from build123d import *

# Parameters (mm, degrees)
BOSS_EXTRUDE1_DEPTH     = 18
SKETCH2_R               = 3.175
CUT_EXTRUDE1_DEPTH      = 1.048172096
CUT_EXTRUDE1_DEPTH_BACK = 29.412494693
FILLET1_R               = 2.54


with BuildPart() as part:
    # Sketch1 → Boss-Extrude1 (new body)
    with BuildSketch(Plane.XY):
        with BuildLine():
            Line((0, -26.9), (25.314659544, -26.9))
            add(Edge.make_bspline(
                [(25.314659544, -26.9), (29.018808902, -26.95946599), (36.438320652, -26.653818936), (47.452273732, -24.92488313), (58.262486614, -21.924318782), (67.016013602, -18.37965694), (73.811742851, -14.890308818), (80.427413207, -11.130302547), (86.897235914, -7.369109823), (93.386399422, -4.327041649), (98.298472606, -2.578666278), (102.47088341, -1.703494583), (105.870866673, -1.428331861), (107.623577227, -1.449984583), (108.491279544, -1.5)],
                knots=[0.000136912, 0.000136912, 0.000136912, 0.000136912, 0.125180551, 0.250224189, 0.375267828, 0.500311467, 0.562833286, 0.625355105, 0.750398744, 0.812920563, 0.875442382, 0.937964202, 0.969225111, 1.000486021, 1.000486021, 1.000486021, 1.000486021], degree=3))
            Line((108.491279544, -1.5), (200, -1.5))
            Line((200, -1.5), (200, 1.5))
            Line((200, 1.5), (108.577128094, 1.5))
            add(Edge.make_bspline(
                [(25.338879667, -23.9), (28.926162088, -23.958039606), (36.111765907, -23.664827946), (46.778323763, -21.99406658), (57.248447209, -19.093410872), (65.732493814, -15.662477543), (72.314760278, -12.28848554), (78.848846724, -8.579093587), (85.394977085, -4.766737379), (92.155894885, -1.585137398), (97.388130608, 0.290112445), (101.932358434, 1.257689935), (105.679869219, 1.570192395), (107.61823033, 1.553901023), (108.577128094, 1.5)],
                knots=[-0.00013852, -0.00013852, -0.00013852, -0.00013852, 0.124820277, 0.249779073, 0.37473787, 0.499696666, 0.562176065, 0.624655463, 0.749614259, 0.812093658, 0.874573056, 0.937052454, 0.968292153, 0.999531852, 0.999531852, 0.999531852, 0.999531852], degree=3))
            Line((25.338879667, -23.9), (0, -23.9))
            Line((0, -23.9), (0, -26.9))
        make_face()
    extrude(amount=BOSS_EXTRUDE1_DEPTH)

    # Sketch2 → Cut-Extrude1 (cut, two sides)
    with BuildSketch(Plane(origin=(0, 1.5, 0), x_dir=(1, 0, 0), z_dir=(0, 1, 0))) as cut_extrude1_sk:
        with Locations((11.847374462, -9)):
            Circle(SKETCH2_R)
        with Locations((180.157387408, -9)):
            Circle(SKETCH2_R)
    extrude(amount=CUT_EXTRUDE1_DEPTH, mode=Mode.SUBTRACT)
    extrude(cut_extrude1_sk.sketch, amount=-CUT_EXTRUDE1_DEPTH_BACK, mode=Mode.SUBTRACT)

    # Fillet1
    fillet1_edges = [part.edges().sort_by_distance(p)[0] for p in [
        (0, -25.4, 0),
        (200, 0, 18),
        (0, -25.4, 18),
        (200, 0, 0),
    ]]
    fillet(fillet1_edges, radius=FILLET1_R)


solid = part.part
The model under review builds one solid part; all positions refer to its coordinate system, in mm. Give positions to 0.01 mm unless a question says otherwise; leave off trailing zeros. Order: outer loops, then holes, each group sorted by start corner. A loop starts at its lowest first (then second) coordinate and runs counter-clockwise, first axis right, second up. Notation, with made-up numbers: (85.5, -5.5) -> (144.5, -5.5) arc R19 cw to (144.5, 24.5) -> close; hole circle Ø6 at (37.25, 32.25). An arc over 180 degrees is marked (long way). Write item = value, one per line. Start each with the question number.
(1) Take a section at A-A (z = 9). State how many separate pieces and enclosed holes the cut face has, plus the area to 3 significant figures.
(2) For L1, parallel to Y at x = 121, z = 15.75; L2, parallel to Y at x = 54.5, z = 14; L3, parallel to X at y = -15.5, z = 10.5, list the stretches that pass through material, from the lowest coordinate up. Write a range as from..to.
(3) Take a section at B-B (x = 146.5). Write out the cut boundary in (y, z).
(4) Draft analysis for pull direction Z (two halves, no side actions). For faces 1 (the flat face through (100, -2, 0)), 2 (the flat face through (154, -1.5, 9)), 3 (the cylindrical face through (9.328, -25.379, 10.932)), state which applies: +Z half, -Z half, draft (parallel to the pull), parting line (faces both ways), or undercut.
(5) For pin 1 Ø1 at (x, z) = (75.5, 11.5) entering from -Y; pin 2 Ø10 at (y, z) = (-13, 13.5) entering from +X; pin 3 Ø8.5 at (x, z) = (180.16, 9) entering from +Y, all flat-tipped, find the tip position at first contact; note any pin that passes through.
Returned:
q1.separate_pieces = 3
q1.enclosed_holes = 0
q1.area = 577 mm²
q2.L1 = -1.5..1.5
q2.L2 = -22.9..-19.76
q2.L3 = 65.78..72.58
q3.outline = (-1.5, 0) -> (1.5, 0) -> (1.5, 18) -> (-1.5, 18) -> close
q4.face_1 = -Z half
q4.face_2 = draft
q4.face_3 = undercut
q5.pin_1 = -14.19
q5.pin_2 = 85.98
q5.pin_3 = 1.5
